Check sheet for the modelled part. Datum: model origin and axes. Units: mm. Face numbers are marked on the shaded views. Coordinates: 2 decimals unless noted, no trailing zeros. Loops run counter-clockwise (first coordinate to the right, second up) from the corner with the lowest first, then second, coordinate; pieces in that order, holes last. Notation, with made-up numbers: M 14,-5 L 72,-5 A26 cw 72,30 Z; hole C -31.5,57.5 d1. An arc over 180 degrees is marked long. Answer as CSV lines item,"result". Start each with the question number.
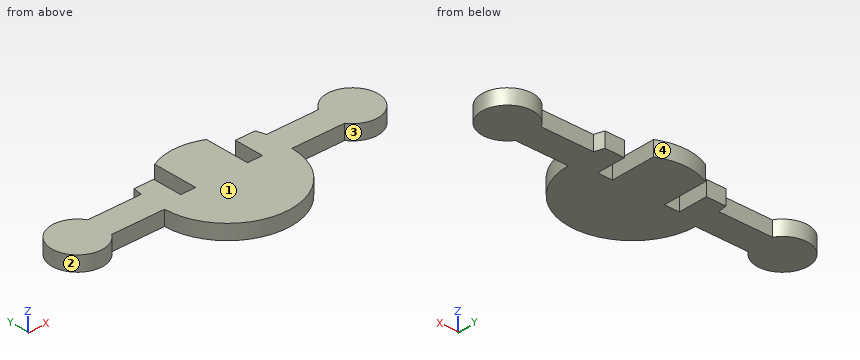
from build123d import *

# Parameters (mm, degrees)
BASE_EXTRUDE_DEPTH = 3


with BuildPart() as part:
    # Sketch1 → Base-Extrude (new body)
    with BuildSketch(Plane.XY):
        with BuildLine():
            Line((380.162891568, 81.023267436), (390.599019838, 81.023267436))
            ThreePointArc((390.599019838, 81.023267436), (400.101534094, 78.637901495), (390.795096715, 75.575554167))
            Line((390.795096715, 75.575554167), (380.207812671, 75.575554167))
            ThreePointArc((380.207812671, 75.575554167), (367.447420728, 62.962928121), (354.687028785, 75.575554167))
            Line((354.687028785, 75.575554167), (344.099744741, 75.575554167))
            ThreePointArc((344.099744741, 75.575554167), (334.793307361, 78.637901495), (344.295821617, 81.023267436))
            Line((344.295821617, 81.023267436), (355.018550657, 81.023267436))
            Line((355.018550657, 81.023267436), (355.321416521, 82.905419895))
            Line((355.321416521, 82.905419895), (359.252420728, 82.905419895))
            Line((359.252420728, 82.905419895), (359.252420728, 77.010044337))
            Line((359.252420728, 77.010044337), (362.252420728, 77.010044337))
            Line((362.252420728, 77.010044337), (362.252420728, 85.966138483))
            ThreePointArc((362.252420728, 85.966138483), (367.447420728, 87.208332237), (372.642420728, 85.966138483))
            Line((372.642420728, 85.966138483), (372.642420728, 77.010044337))
            Line((372.642420728, 77.010044337), (375.642420728, 77.010044337))
            Line((375.642420728, 77.010044337), (375.642420728, 82.905419895))
            Line((375.642420728, 82.905419895), (379.573424935, 82.905419895))
            Line((379.573424935, 82.905419895), (380.162891568, 81.023267436))
        make_face()
    extrude(amount=BASE_EXTRUDE_DEPTH)


solid = part.part
Item 1: Sectioned sample at B-B, the plane z = 1.35. Record the boundary of the cut face in (x, y).
Item 2: Sectioned sample at C-C, the plane x = 382.5. Record the boundary of the cut face in (y, z).
Item 3: Go/stop test with flat-tipped pins: pin 1 (0.9 mm diameter, centred on y = 83, z = 1, fed in from -X); pin 2 (1.5 mm diameter, centred on y = 74.5, z = 1, fed in from +X); pin 3 (1.5 mm diameter, centred on x = 374.5, z = 2, fed in from +Y); pin 4 (5 mm diameter, centred on x = 393.5, y = 76, fed in from -Z). Record where each tip stops, or that it passes through.
Item 4: Sectioned sample at A-A, the plane y = 74. Record the boundary of the cut face in (x, z).
Item 5: Release check for a two-part mould opening along X. For the marked faces 1, 2, 3 and 4 record: released by +X, released by -X, zero draft, split by the parting line, or undercut.
Item 6: Material ranges on line 1 (X direction, y = 78.25, z = 2.9); line 2 (X direction, y = 81.25, z = 2.1); line 3 (X direction, y = 75, z = 0.8), recorded low to high. Write a range as from..to.
Item 7: Sectioned sample at D-D, the plane y = 79.75. Record the boundary of the cut face in (x, z).
Reply:
1,outline,"M 344.1,75.58 L 354.69,75.58 A12.76 ccw 380.21,75.58 L 390.8,75.58 A5.1 ccw long 390.6,81.02 L 380.16,81.02 L 379.57,82.91 L 375.64,82.91 L 375.64,77.01 L 372.64,77.01 L 372.64,85.97 A11.48 ccw 362.25,85.97 L 362.25,77.01 L 359.25,77.01 L 359.25,82.91 L 355.32,82.91 L 355.02,81.02 L 344.3,81.02 A5.1 ccw long Z"
2,outline,"M 75.58,0 L 81.02,0 L 81.02,3 L 75.58,3 Z"
3,pin 1,"x = 336.85"
3,pin 2,"x = 398.97"
3,pin 3,"y = 77.01"
3,pin 4,"z = 0"
4,outline,"M 337.41,0 L 342.37,0 L 342.37,3 L 337.41,3 Z; M 354.8,0 L 380.09,0 L 380.09,3 L 354.8,3 Z; M 392.52,0 L 397.49,0 L 397.49,3 L 392.52,3 Z"
5,face 1,"zero draft"
5,face 2,"undercut"
5,face 3,"undercut"
5,face 4,"split by the parting line"
6,line 1,"334.79..359.25, 362.25..372.64, 375.64..400.1"
6,line 2,"335.62..344.16, 355.06..359.25, 362.25..372.64, 375.64..380.09, 390.74..399.27"
6,line 3,"336.14..343.64, 354.71..380.19, 391.25..398.76"
7,outline,"M 334.96,0 L 359.25,0 L 359.25,3 L 334.96,3 Z; M 362.25,0 L 372.64,0 L 372.64,3 L 362.25,3 Z; M 375.64,0 L 399.94,0 L 399.94,3 L 375.64,3 Z"
